from build123d import *

# Parameters (mm, degrees)
BOSS_EXTRUDE1_DEPTH = 1.6
BOSS_EXTRUDE2_DEPTH = 1.6


with BuildPart() as part:
    # Sketch1 → Boss-Extrude1 (new body)
    with BuildSketch(Plane.XY):
        Polygon((0, 20.012034266), (-1.403252859, 21.209327608), (-5.593180392, 3.61901348), (-5.013506757, 3.124420236), (-7.321608561, 0.419276606), (-19.784591715, 11.053031347), (-17.476489911, 13.758174978), (-16.896816276, 13.263581734), (-2.176151039, 21.868785266), (-3.680398963, 23.152250331), (-25.4, 23.152250331), (-25.4, -3.81), (0, -3.81), align=None)
    extrude(amount=BOSS_EXTRUDE1_DEPTH)

    # Sketch2 → Boss-Extrude2 (add)
    with BuildSketch(Plane.XY.offset(1.6)):
        Polygon((-19.524962716, 11.357321969), (-7.061979562, 0.723567228), (-7.321608561, 0.419276606), (-19.784591715, 11.053031347), align=None)
    extrude(amount=-BOSS_EXTRUDE2_DEPTH)


solid = part.part
For this review, take the finished solid that the model builds, in its own axes (mm). A direction names the side the tool comes from. Round coordinates to 2 decimals unless told otherwise and drop trailing zeros. Loops run counter-clockwise (first coordinate to the right, second up) from the corner with the lowest first, then second, coordinate; pieces in that order, holes last. Notation, with made-up numbers: (26, 33.5) - (49, 33.5) arc R12 ccw to (49, 49.5) - close; hole circle Ø10 at (35.5, 76.25). An arc over 180 degrees is marked (long way). One line per item, written item: value. Start each with the question number.
Item 1: For faces 1 (the flat face through (-25.4, 10, 1)), 2 (the flat face through (-13.381, 6.115, 0.811)), list the 3-axis set-ups (+Z, -Z, +X, -X, +Y, -Y) from which the entire face can be reached by the end or side of a thin tool; tool diameter is ignored.
Item 2: The part is to be moulded in two halves that separate along X. For faces 3 (the flat face through (-15, 7, 0)), 4 (the flat face through (-9.64, 17.506, 0.789)), 5 (the flat face through (-0.69, 20.6, 0.79)), say which applies: +X half, -X half, draft (parallel to the pull), parting line (faces both ways), or undercut.
Item 3: For L1, parallel to X at y = 4.75, z = 1.55; L2, parallel to X at y = 20, z = 0.35; L3, parallel to X at y = 13.5, z = 1.45, list the stretches that pass through material, from the lowest coordinate up.
Item 4: Take a section at B-B (z = 0.35). Give the boundary of the cut face in (x, y), plus the area to 3 significant figures.
Item 5: Take a section at A-A (y = 7.5). Give the boundary of the cut face in (x, z), plus the area to 3 significant figures.
Item 6: Take a section at C-C (x = -3). Give the boundary of the cut face in (y, z), plus the area to 3 significant figures.
Answer below:
1. face 1: +Z, -Z, -X, +Y, -Y
1. face 2: +Z, -Z
2. face 3: draft
2. face 4: undercut
2. face 5: +X half
3. L1: x = -25.4 to -11.78, -5.32 to 0
3. L2: x = -25.4 to -5.37, -1.69 to 0
3. L3: x = -25.4 to -17.7, -17.17 to -16.49, -3.24 to 0
4. outline: (-25.4, -3.81) - (0, -3.81) - (0, 20.01) - (-1.4, 21.21) - (-5.59, 3.62) - (-5.01, 3.12) - (-7.06, 0.72) - (-19.52, 11.36) - (-17.48, 13.76) - (-16.9, 13.26) - (-2.18, 21.87) - (-3.68, 23.15) - (-25.4, 23.15) - close
4. area: 500 mm2
5. outline: (-25.4, 0) - (-15, 0) - (-15, 1.6) - (-25.4, 1.6) - close; (-4.67, 0) - (0, 0) - (0, 1.6) - (-4.67, 1.6) - close
5. area: 24.1 mm2
6. outline: (-3.81, 0) - (14.51, 0) - (14.51, 1.6) - (-3.81, 1.6) - close; (21.39, 0) - (22.57, 0) - (22.57, 1.6) - (21.39, 1.6) - close
6. area: 31.2 mm2
